Read the model definition and answer for the solid it produces. Units are mm, in the model's axes. Face numbers are marked on the shaded views. A direction names the side the tool comes from. Round coordinates to 2 decimals unless told otherwise and drop trailing zeros. Order: outer loops, then holes, each group sorted by start corner. A loop starts at its lowest first (then second) coordinate and runs counter-clockwise, first axis right, second up. Notation, with made-up numbers: (12.5, -38.75) -> (39.5, -38.75) arc R29 ccw to (39.5, 0.25) -> close; hole circle Ø10 at (29, -10). An arc over 180 degrees is marked (long way). Answer as a JSON object with one key per item and string values. Group by question number.
Item 1: Section D-D, the plane z = -15.4 is taken. Write down the section's boundary in (x, y) (3 decimals).
Item 2: Section B-B, the plane y = 8 is taken. Write down the section's boundary in (x, z) (3 decimals).
Item 3: Section C-C, the plane x = -10 is taken. Write down the section's boundary in (y, z) (3 decimals), plus the area to 3 significant figures.
Item 4: Consider probe 1 along X at (y, z) = (6.5, 15); probe 2 along Z at (x, y) = (11, 5.5); probe 3 along Z at (x, y) = (4, -0.25). Determine where each line is inside the solid, lowest interval first. Write a range as from..to.
Item 5: Section A-A, the plane y = -3.25 is taken. Write down the section's boundary in (x, z), plus the area to 3 significant figures.
Item 6: The mould has two halves that part along X. Classify the marked faces 1, 2 and 3: pulls with the +X half, pulls with the -X half, needs draft (parallel to the pull), parting line crosses it, or undercut.
Item 7: For the marked faces 4, 5, 6 and 7, determine the directions among +Z, -Z, +X, -X, +Y, -Y from which every point of the face is accessible in a straight line to the end or side of a thin tool.
Item 8: Given P1, Ø3, axis at x = 5, z = 14.5, coming from the -Y side; P2, Ø5, axis at x = 2, z = 12, coming from the +Y side; P3, Ø4, axis at x = -3, y = -3, coming from the -Z side, each flat-ended and moving along its own axis, determine where each tip first touches the part or whether it passes through.
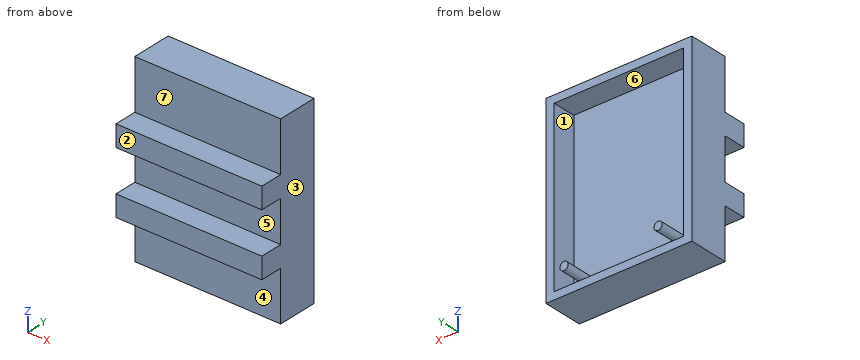
from build123d import *

# Parameters (mm, degrees)
SKETCH1_W           = 31
SKETCH1_H           = 39
BOSS_EXTRUDE1_DEPTH = 8.5
SKETCH5_W           = 31
SKETCH5_H           = 4.5
BOSS_EXTRUDE3_DEPTH = 4.8
SKETCH7_W           = 27.5
SKETCH7_H           = 35.8
CUT_EXTRUDE1_DEPTH  = 5
SKETCH8_R           = 0.875
BOSS_EXTRUDE4_DEPTH = 7


with BuildPart() as part:
    # Sketch1 → Boss-Extrude1 (new body)
    with BuildSketch(Plane(origin=(0, 0, 0), x_dir=(1, 0, 0), z_dir=(0, 1, 0))):
        Rectangle(SKETCH1_W, SKETCH1_H)
    extrude(amount=BOSS_EXTRUDE1_DEPTH)

    # Sketch5 → Boss-Extrude3 (add)
    with BuildSketch(Plane.XZ):
        with Locations((0, 6.65)):
            Rectangle(SKETCH5_W, SKETCH5_H)
    boss_extrude3 = extrude(amount=BOSS_EXTRUDE3_DEPTH)

    # Mirror1: Boss-Extrude3 across plane
    add(boss_extrude3.mirror(Plane.XY))

    # Sketch7 → Cut-Extrude1 (cut)
    with BuildSketch(Plane(origin=(0, 8.5, 0), x_dir=(1, 0, 0), z_dir=(0, 1, 0))):
        Rectangle(SKETCH7_W, SKETCH7_H)
    extrude(amount=-CUT_EXTRUDE1_DEPTH, mode=Mode.SUBTRACT)

    # Sketch8 → Boss-Extrude4 (add)
    with BuildSketch(Plane(origin=(0, 3.5, 0), x_dir=(1, 0, 0), z_dir=(0, 1, 0))):
        with Locations(Location((-10, 15.4, 0), (0, 0, 90))):
            Circle(SKETCH8_R)
        with Locations(Location((10, 15.4, 0), (0, 0, 90))):
            Circle(SKETCH8_R)
    extrude(amount=BOSS_EXTRUDE4_DEPTH)


solid = part.part
Values found:
{
 "1": {"outline": "(-15.5, 0) -> (15.5, 0) -> (15.5, 8.5) -> (13.75, 8.5) -> (13.75, 3.5) -> (10.875, 3.5) -> (10.875, 10.5) -> (9.125, 10.5) -> (9.125, 3.5) -> (-9.125, 3.5) -> (-9.125, 10.5) -> (-10.875, 10.5) -> (-10.875, 3.5) -> (-13.75, 3.5) -> (-13.75, 8.5) -> (-15.5, 8.5) -> close"},
 "2": {"outline": "(-15.5, -19.5) -> (15.5, -19.5) -> (15.5, 19.5) -> (-15.5, 19.5) -> close; circle Ø1.75 at (-10, -15.4); circle Ø1.75 at (10, -15.4); hole (-13.75, -17.9) -> (13.75, -17.9) -> (13.75, 17.9) -> (-13.75, 17.9) -> close"},
 "3": {"outline": "(-4.8, -8.9) -> (0, -8.9) -> (0, -19.5) -> (8.5, -19.5) -> (8.5, -17.9) -> (3.5, -17.9) -> (3.5, -16.275) -> (10.5, -16.275) -> (10.5, -14.525) -> (3.5, -14.525) -> (3.5, 17.9) -> (8.5, 17.9) -> (8.5, 19.5) -> (0, 19.5) -> (0, 8.9) -> (-4.8, 8.9) -> (-4.8, 4.4) -> (0, 4.4) -> (0, -4.4) -> (-4.8, -4.4) -> close", "area": "208 mm2"},
 "4": {"probe 1": "-15.5..-13.75, 13.75..15.5", "probe 2": "-19.5..-17.9, 17.9..19.5", "probe 3": "-8.9..-4.4, 4.4..8.9"},
 "5": {"outline": "(-15.5, -8.9) -> (15.5, -8.9) -> (15.5, -4.4) -> (-15.5, -4.4) -> close; (-15.5, 4.4) -> (15.5, 4.4) -> (15.5, 8.9) -> (-15.5, 8.9) -> close", "area": "279 mm2"},
 "6": {"face 1": "undercut", "face 2": "needs draft", "face 3": "pulls with the +X half"},
 "7": {"face 4": "-Z, +X, -X, -Y", "face 5": "+X, -X, -Y", "face 6": "+Y", "face 7": "+Z, +X, -X, -Y"},
 "8": {"P1": "y = 0", "P2": "y = 3.5", "P3": "z = -8.9"}
}
